Source: CAD feature listing. Evaluate the final solid. Frame: model axes, mm. A direction names the side the tool comes from. Give positions to 0.01 mm unless a question says otherwise; leave off trailing zeros. Order: outer loops, then holes, each group sorted by start corner. A loop starts at its lowest first (then second) coordinate and runs counter-clockwise, first axis right, second up.
```python
from build123d import *

# Parameters (mm, degrees)
F0_R        = 1.65
F1_DEPTH    = 5
F2_T1_DEPTH = 5
F3_T1_DEPTH = 5


# Not quite as in the source:
# - a fillet or chamfer that OpenCascade refuses, or shapes differently, is made with other operations: its cross-section is extruded or revolved along the edge and cut away or added


with BuildPart() as f1:
    # F0 (on Top) → F1 (new body)
    with BuildSketch(Plane.XY):
        Polygon((7.0434366612, 0), (14.0868733224, 0), (17.9254915565, 0), (17.9254915565, 12.1765555814), (17.9254915565, 13.6025686192), align=None)
        Polygon((0, 0), (7.0434366612, 0), (17.9254915565, 13.6025686192), (17.9254915565, 17.9254915565), (7.296956584, 17.9254915565), (0, 8.8042958265), align=None)
        with Locations((15.25, 15.25)):
            Circle(F0_R, mode=Mode.SUBTRACT)
        with BuildLine():
            Line((17.9254915565, 17.9254915565), (17.9254915565, 13.6025686192))
            Line((17.9254915565, 13.6025686192), (17.9254915565, 12.1765555814))
            Line((17.9254915565, 12.1765555814), (20, 12.1765555814))
            Line((20, 12.1765555814), (23.3218736491, 20.3480462349))
            Line((23.3218736491, 20.3480462349), (97.8522087861, 113.5109651562))
            ThreePointArc((97.8522087861, 113.5109651562), (92.8542693342, 116.0678366678), (89.2626518823, 120.3826106793))
            Line((89.2626518823, 120.3826106793), (7.296956584, 17.9254915565))
            Line((7.296956584, 17.9254915565), (17.9254915565, 17.9254915565))
        make_face()
        with Locations((20, 20)):
            Circle(F0_R, mode=Mode.SUBTRACT)
        Polygon((0, 17.9254915565), (0, 8.8042958265), (7.296956584, 17.9254915565), align=None)
        with BuildLine():
            ThreePointArc((106.0792785003, 140.2640892683), (90.9109583101, 136.0412602966), (89.2626518823, 120.3826106793))
            ThreePointArc((89.2626518823, 120.3826106793), (92.8542693342, 116.0678366678), (97.8522087861, 113.5109651562))
            ThreePointArc((97.8522087861, 113.5109651562), (112.7671167579, 118.5563335383), (113.5573186397, 134.2816571567))
            Line((113.5573186397, 134.2816571567), (107.5786593199, 130.6408285784))
            Line((107.5786593199, 130.6408285784), (103.8396392501, 133.6320446341))
            Line((103.8396392501, 133.6320446341), (106.0792785003, 140.2640892683))
        make_face()
    extrude(amount=F1_DEPTH)

    # F2: fillet of radius 3 on 6 edges, made by hand

    # F2_s2 → F2_t1 (join)
    with BuildSketch(Plane.XY):
        with BuildLine():
            ThreePointArc((8.1976884699, 19.0514064139), (7.1546482331, 18.2215818476), (5.8550820416, 17.9254915565))
            Line((5.8550820416, 17.9254915565), (7.296956584, 17.9254915565))
            Line((7.296956584, 17.9254915565), (8.1976884699, 19.0514064139))
        make_face()
        with BuildLine():
            ThreePointArc((17.9254915565, 9.3228798152), (18.4989225106, 11.0868987111), (20, 12.1765555814))
            Line((20, 12.1765555814), (17.9254915565, 12.1765555814))
            Line((17.9254915565, 12.1765555814), (17.9254915565, 9.3228798152))
        make_face()
        with BuildLine():
            ThreePointArc((96.6977481783, 112.0678893964), (97.9486405, 112.9881128103), (99.4920567349, 113.1596035031))
            ThreePointArc((99.4920567349, 113.1596035031), (98.6668668075, 113.3107074808), (97.8522087861, 113.5109651562))
            Line((97.8522087861, 113.5109651562), (96.6977481783, 112.0678893964))
        make_face()
        with BuildLine():
            ThreePointArc((88.5598934027, 121.9053341689), (88.7313840955, 120.361917934), (88.1081912745, 118.9395349195))
            Line((88.1081912745, 118.9395349195), (89.2626518823, 120.3826106793))
            ThreePointArc((89.2626518823, 120.3826106793), (88.8884511699, 121.1334399909), (88.5598934027, 121.9053341689))
        make_face()
        with BuildLine():
            ThreePointArc((105.4799499303, 132.31979609), (104.4752105502, 133.8183827512), (104.5117302298, 135.6222479112))
            Line((104.5117302298, 135.6222479112), (103.8396392501, 133.6320446341))
            Line((103.8396392501, 133.6320446341), (105.4799499303, 132.31979609))
        make_face()
        with BuildLine():
            ThreePointArc((109.3727888874, 131.7334009852), (107.6209369535, 131.3018016285), (105.9383486397, 131.9530771225))
            Line((105.9383486397, 131.9530771225), (107.5786593199, 130.6408285784))
            Line((107.5786593199, 130.6408285784), (109.3727888874, 131.7334009852))
        make_face()
    extrude(amount=F2_T1_DEPTH)

    # F3: fillet of radius 199.9181440352 on 1 edges, made by hand

    # F3_s2 → F3_t1 (join)
    with BuildSketch(Plane.XY):
        with BuildLine():
            ThreePointArc((20, 12.1765555814), (28.3645778619, 25.6450570093), (37.770134119, 38.4083718223))
            Line((37.770134119, 38.4083718223), (23.3218736491, 20.3480462349))
            Line((23.3218736491, 20.3480462349), (20, 12.1765555814))
        make_face()
    extrude(amount=F3_T1_DEPTH)

    # F4: F1 across plane


with BuildPart() as f1_1:
    add(f1.part)
    add(f1.part.mirror(Plane.YZ))

    # F5: F1 across plane


with BuildPart() as f1_2:
    add(f1_1.part)
    add(f1_1.part.mirror(Plane.XZ))


solid = f1_2.part
```
1) Section query A-A, the plane y = -27. Return the cut outline in (x, z), and give its area (3 significant figures).
Report:
outline: (-29.29, 0) - (-14.56, 0) - (-14.56, 5) - (-29.29, 5) - close; (14.56, 0) - (29.29, 0) - (29.29, 5) - (14.56, 5) - close
area: 147 mm2
2) Draft query along X for faces 4 (the cylindrical face through (-28.24, -25.46, 2.46)), 5 (the cylindrical face through (91.6, 136.8, 2.5)), 6 (the cylindrical face through (28.24, 25.46, 2.46)), 7 (the flat face through (9, 10, 5)). Return one class per face: +X half, -X half, draft (parallel to the pull), parting line (faces both ways), or undercut.
Report:
face 4: -X half
face 5: undercut
face 6: +X half
face 7: draft
3) Section query C-C, the plane z = 3.8. Count the separate pieces of the cut face and the enclosed holes in it, and give its area (3 significant figures).
Report:
separate pieces: 1
enclosed holes: 8
area: 9,180 mm2
4) Pin query (flat end, axial travel): pin 1 (5.5 mm diameter, centred on x = 15.25, y = -15.25, fed in from -Z); pin 2 (2.5 mm diameter, centred on x = 2.5, z = 1.5, fed in from +Y); pin 3 (1.5 mm diameter, centred on x = 74, z = 3, fed in from +Y); pin 4 (2 mm diameter, centred on y = 103, z = 3, fed in from +X). Return the tip coordinate at first contact, or that it passes through.
Report:
pin 1: stops at z = 0
pin 2: stops at y = 17.93
pin 3: stops at y = 102.24
pin 4: stops at x = 90.24
5) Material intervals for L1, parallel to Y at x = -15.25, z = 3.5; L2, parallel to Y at x = -14, z = 3.7; L3, parallel to Y at x = 2.5, z = 3.35, sorted ascending.
Report:
L1: y = -27.87 to -16.9, -13.6 to 13.6, 16.9 to 27.87
L2: y = -26.3 to -16.33, -14.17 to 14.17, 16.33 to 26.3
L3: y = -17.93 to 17.93
6) Reachability of faces 1 (the flat face through (66.82, 74.72, 2.46)), 2 (the flat face through (9, 10, 0)), 3 (the flat face through (-66.82, -74.72, 2.46)) from +Z, -Z, +X, -X, +Y, -Y: full face, straight path, thin tool, end or side. Return the list, or none.
Report:
face 1: +Z, -Z, +X
face 2: -Z, +X, -X, +Y, -Y
face 3: +Z, -Z, -X
7) Section query B-B, the plane x = 56.5. Return the cut outline in (y, z), and give its area (3 significant figures).
Report:
outline: (-79.43, 0) - (-61.82, 0) - (-61.82, 5) - (-79.43, 5) - close; (61.82, 0) - (79.43, 0) - (79.43, 5) - (61.82, 5) - close
area: 176 mm2
